Part model, mm, in its own coordinate system. Face numbers are marked on the shaded views. Give positions to 0.01 mm unless a question says otherwise; leave off trailing zeros. Write each loop counter-clockwise with the first axis right and the second up, starting at its lowest first coordinate (ties: lowest second). Pieces come first, ordered by that corner, then holes. Notation, with made-up numbers: M -13,-7.75 L -6,-7.75 A6 cw -6,0.25 Z; hole C -26.75,-37 d9. An arc over 180 degrees is marked long. Answer as CSV lines item,"result". Start each with the question number.
1) Slice it at B-B, the plane z = 2.1. Give the cut face in (x, y).
2) Slice it at C-C, the plane x = 125. Give the cut face in (y, z), plus the area to 3 significant figures.
3) Mould opens along X. For the marked faces 1, 2 and 3 say: pulls with the +X half, pulls with the -X half, needs draft (parallel to the pull), parting line crosses it, or undercut.
4) Slice it at A-A, the plane y = 10. Give the cut face in (x, z).
5) Wall check: line 1 along X through (y, z) = (1.5, 2.35); line 2 along Y through (x, z) = (127.25, 1.15); line 3 along X through (y, z) = (8.25, 0.1). Give the ranges that are in metal, low to high. Write a range as from..to.
6) Pin check, flat tips, straight feed: pin 1 Ø2.5 at (x, y) = (132.86, 9.07) entering from -Z; pin 2 Ø5 at (x, y) = (114, 9.5) entering from -Z; pin 3 Ø1 at (x, z) = (135.5, 2) entering from +Y. Stop position of each tip, or through.
7) Slice it at D-D, the plane y = 0. Give the cut face in (x, z).
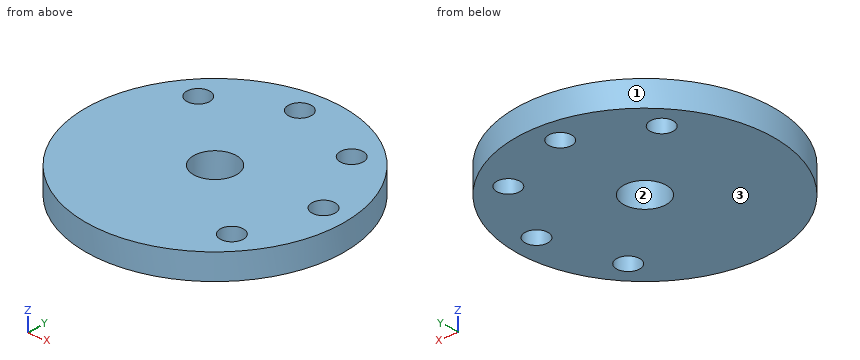
```python
from build123d import *

# Parameters (mm, degrees)
SKETCH_1_R      = 15
SKETCH_1_R_2    = 1.35
SKETCH_1_R_3    = 2.5
EXTRUDE_1_DEPTH = 3


with BuildPart() as part:
    # 草图1 → 凸台-拉伸1 (new body)
    with BuildSketch(Plane.XY):
        with Locations((125, 0)):
            Circle(SKETCH_1_R)
        with Locations((132.860147625, 9.067418558)):
            Circle(SKETCH_1_R_2, mode=Mode.SUBTRACT)
        with Locations((136.969596837, 0.853669463)):
            Circle(SKETCH_1_R_2, mode=Mode.SUBTRACT)
        with Locations((134.067418558, -7.860147625)):
            Circle(SKETCH_1_R_2, mode=Mode.SUBTRACT)
        with Locations((124.146330537, 11.969596837)):
            Circle(SKETCH_1_R_2, mode=Mode.SUBTRACT)
        with Locations((115.932581442, 7.860147625)):
            Circle(SKETCH_1_R_2, mode=Mode.SUBTRACT)
        with Locations((125, 0)):
            Circle(SKETCH_1_R_3, mode=Mode.SUBTRACT)
    extrude(amount=EXTRUDE_1_DEPTH)


solid = part.part
```
Found:
1,outline,"C 125,0 d30; hole C 115.93,7.86 d2.7; hole C 125,0 d5; hole C 124.15,11.97 d2.7; hole C 132.86,9.07 d2.7; hole C 134.07,-7.86 d2.7; hole C 136.97,0.85 d2.7"
2,outline,"M -15,0 L -2.5,0 L -2.5,3 L -15,3 Z; M 2.5,0 L 10.92,0 L 10.92,3 L 2.5,3 Z; M 13.02,0 L 15,0 L 15,3 L 13.02,3 Z"
2,area,"68.7 mm²"
3,face 1,"parting line crosses it"
3,face 2,"undercut"
3,face 3,"needs draft"
4,outline,"M 113.82,0 L 131.88,0 L 131.88,3 L 113.82,3 Z; M 133.84,0 L 136.18,0 L 136.18,3 L 133.84,3 Z"
5,line 1,"110.08..123, 127..135.78, 138.15..139.92"
5,line 2,"-14.83..-1.09, 1.09..14.83"
5,line 3,"112.47..114.64, 117.23..131.79, 133.93..137.53"
6,pin 1,"through"
6,pin 2,"z = 0"
6,pin 3,"y = 11.18"
7,outline,"M 110,0 L 122.5,0 L 122.5,3 L 110,3 Z; M 127.5,0 L 135.92,0 L 135.92,3 L 127.5,3 Z; M 138.02,0 L 140,0 L 140,3 L 138.02,3 Z"
